from build123d import *

# Parameters (mm, degrees)
SKETCH1_W                      = 38.1
SKETCH1_H                      = 38.1
SKETCH1_W_2                    = 114.3
BOSS_EXTRUDE1_DEPTH            = 6.35
F_5_16_0_3125_DIAMETER_HOLE1_D = 7.9375


with BuildPart() as part:
    # Sketch1 → Boss-Extrude1 (new body)
    # profile 1 of 3: a face of its own
    with BuildSketch(Plane.XY):
        Polygon((152.4, 0), (0, 0), (0, 76.2), (38.1, 146.05), (114.3, 146.05), (152.4, 76.2), align=None)
        with Locations((76.2, 107.95)):
            Rectangle(SKETCH1_W, SKETCH1_H, mode=Mode.SUBTRACT)
        with Locations((76.2, 38.1)):
            Rectangle(SKETCH1_W_2, SKETCH1_H, mode=Mode.SUBTRACT)
    # profile 2 of 3: a face of its own
    with BuildSketch(Plane.XY):
        with Locations((76.2, 107.95)):
            Rectangle(SKETCH1_W, SKETCH1_H)
    # profile 3 of 3: a face of its own
    with BuildSketch(Plane.XY):
        with Locations((76.2, 38.1)):
            Rectangle(SKETCH1_W_2, SKETCH1_H)
    extrude(amount=BOSS_EXTRUDE1_DEPTH)

    # 5/16 (0.3125) Diameter Hole1 (through all)
    with Locations(Plane.XY.offset(6.35)):
        with Locations((19.05, 19.05), (19.05, 57.15), (57.15, 88.9), (57.15, 127), (95.25, 127), (95.25, 88.9), (133.35, 57.15), (133.35, 19.05)):
            Hole(F_5_16_0_3125_DIAMETER_HOLE1_D / 2)


solid = part.part
Build history of the part. All positions in model axes, mm. Round coordinates to 2 decimals unless told otherwise and drop trailing zeros. Write each loop counter-clockwise with the first axis right and the second up, starting at its lowest first coordinate (ties: lowest second). Pieces come first, ordered by that corner, then holes. Notation, with made-up numbers: M 32,57.5 L 41,57.5 A28 cw 41,92.5 Z; hole C 38,3.25 d10. An arc over 180 degrees is marked long. Answer in a Markdown table with one row per item.
1. Saw through at A-A (x = 95.25). List the corners of the cut face in (y, z).
Geometry check:
| item | result |
|---|---|
| outline | M 0,0 L 84.93,0 L 84.93,6.35 L 0,6.35 Z; M 92.87,0 L 123.03,0 L 123.03,6.35 L 92.87,6.35 Z; M 130.97,0 L 146.05,0 L 146.05,6.35 L 130.97,6.35 Z |
2. Flat gauge pin, fed straight in: P1, Ø2, axis at x = 135.5, z = 2, coming from the -Y side. Where does the tip first touch, or does it go through?
Geometry check:
| item | result |
|---|---|
| P1 | y = 0 |
3. Mould opens along X. For faces 1 (the face through (77, 0, 3)), 2 (the face through (137.315, 19.224, 3.131)), 3 (the face through (133.083, 111.614, 3.131)) say: +X half, -X half, draft (parallel to the pull), parting line (faces both ways), or undercut.
Geometry check:
| item | result |
|---|---|
| face 1 | draft |
| face 2 | undercut |
| face 3 | +X half |
4. Probe L1, parallel to Y at x = 57.15, z = 3.75; L2, parallel to X at y = 16, z = 1.25; L3, parallel to Y at x = 131, z = 3.75. List the from-to ranges inside material, lowest first. Write a range as [from, to].
Geometry check:
| item | result |
|---|---|
| L1 | [0, 84.93], [92.87, 123.03], [130.97, 146.05] |
| L2 | [0, 16.51], [21.59, 130.81], [135.89, 152.4] |
| L3 | [0, 15.85], [22.25, 53.95], [60.35, 115.43] |
5. Saw through at C-C (y = 19.05). List the corners of the cut face in (x, z).
Geometry check:
| item | result |
|---|---|
| outline | M 0,0 L 15.08,0 L 15.08,6.35 L 0,6.35 Z; M 23.02,0 L 129.38,0 L 129.38,6.35 L 23.02,6.35 Z; M 137.32,0 L 152.4,0 L 152.4,6.35 L 137.32,6.35 Z |
6. Saw through at D-D (x = 119). List the corners of the cut face in (y, z), and give its area (3 significant figures).
Geometry check:
| item | result |
|---|---|
| outline | M 0,0 L 137.43,0 L 137.43,6.35 L 0,6.35 Z |
| area | 873 mm2 |
7. Saw through at B-B (z = 2.25). State how many separate pieces and enclosed holes the cut face has, and give its area (3 significant figures).
Geometry check:
| item | result |
|---|---|
| separate pieces | 1 |
| enclosed holes | 8 |
| area | 19,200 mm2 |
